The model under review builds one solid part; all positions refer to its coordinate system, in mm. Round coordinates to 2 decimals unless told otherwise and drop trailing zeros. Loops run counter-clockwise (first coordinate to the right, second up) from the corner with the lowest first, then second, coordinate; pieces in that order, holes last. Notation, with made-up numbers: (-38, 21) -> (4, 21) arc R8 ccw to (4, 28) -> close; hole circle Ø6 at (56, 28). An arc over 180 degrees is marked (long way). Write each question's results on one line, items separated by ' | '. Start each with the question number.
Item 1: We need section A-A (z = 13.25). Give the boundary of the cut face in (x, y), and give its area (3 significant figures).
Item 2: For L1, parallel to Z at x = 0.75, y = 12.9; L2, parallel to Y at x = 0.1, z = 7.5; L3, parallel to Y at x = 1.45, z = 0.75, list the stretches that pass through material, from the lowest coordinate up. Write a range as from..to.
Item 3: Mouldability with a two-part tool opening along X and no side actions: class faces 1 (the flat face through (0, 12.4, 0)), 2 (the flat face through (-2, 12.4, 6.9)), 3 (the cylindrical face through (0, 12, 7)), 4 (the flat face through (2, 12.3, 6.9)) as pulls with the +X half, pulls with the -X half, needs draft (parallel to the pull), parting line crosses it, or undercut.
from build123d import *

# Parameters (mm, degrees)
BOSS_EXTRUDE1_DEPTH = 14
FILLET1_R           = 0.1


with BuildPart() as part:
    # Sketch1 → Boss-Extrude1 (new body)
    with BuildSketch(Plane.XY):
        with BuildLine():
            Line((2, 11.832159566), (2, 12.845232579))
            ThreePointArc((2, 12.845232579), (0, 13), (-2, 12.845232579))
            Line((-2, 12.845232579), (-2, 11.832159566))
            ThreePointArc((-2, 11.832159566), (0, 12), (2, 11.832159566))
        make_face()
    extrude(amount=BOSS_EXTRUDE1_DEPTH)

    # Fillet1
    fillet1_edges = [part.edges().sort_by_distance(p)[0] for p in [
        (0, 13, 14),
        (-2, 12.338696072, 14),
        (0, 12, 14),
        (-2, 12.338696072, 0),
        (0, 13, 0),
        (2, 12.338696072, 0),
        (0, 12, 0),
        (2, 12.338696072, 14),
        (-2, 11.832159566, 7),
        (-2, 12.845232579, 7),
        (2, 12.845232579, 7),
        (2, 11.832159566, 7),
    ]]
    fillet(fillet1_edges, radius=FILLET1_R)


solid = part.part
Here are the results:
1) outline: (-2, 11.95) arc R0.1 ccw to (-1.88, 11.85) arc R12 cw to (1.88, 11.85) arc R0.1 ccw to (2, 11.95) -> (2, 12.76) arc R0.1 ccw to (1.91, 12.86) arc R13 ccw to (-1.91, 12.86) arc R0.1 ccw to (-2, 12.76) -> close | area: 4.01 mm2
2) L1: z = 0..14 | L2: y = 12..13 | L3: y = 11.91..12.92
3) face 1: needs draft | face 2: pulls with the -X half | face 3: undercut | face 4: pulls with the +X half
